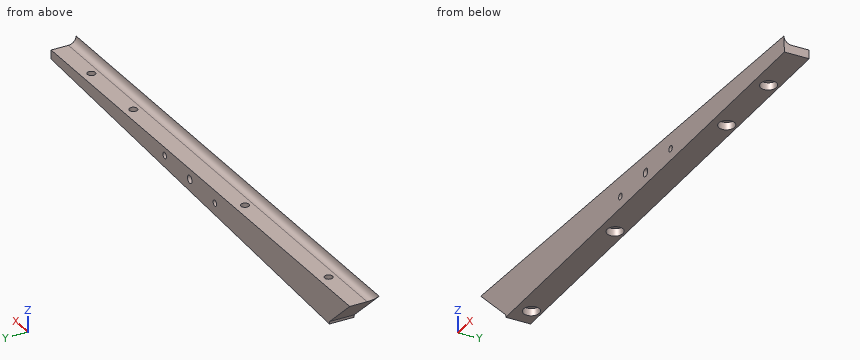
from build123d import *

# Parameters (mm, degrees)
CYLINDER033_R             = 1.6
CYLINDER033_DEPTH         = 100
CYLINDER034_R             = 1.25
CYLINDER034_DEPTH         = 100
CYLINDER035_R             = 1.25
CYLINDER035_DEPTH         = 100
FUSION027_PLACEMENT_ANGLE = 3.00002
CYLINDER012_R             = 3.2
CYLINDER012_DEPTH         = 3
CYLINDER013_R             = 1.6
CYLINDER013_DEPTH         = 30
CYLINDER014_R             = 3.2
CYLINDER014_DEPTH         = 3
CYLINDER015_R             = 1.6
CYLINDER015_DEPTH         = 30
CYLINDER016_R             = 3.2
CYLINDER016_DEPTH         = 3
CYLINDER017_R             = 1.6
CYLINDER017_DEPTH         = 30
CYLINDER011_R             = 3.2
CYLINDER011_DEPTH         = 3
CYLINDER010_R             = 1.6
CYLINDER010_DEPTH         = 30
BOX_W                     = 600
BOX_H                     = 10
BOX_DEPTH                 = 20
BOX_PLACEMENT_ANGLE       = 3
BOX001_W                  = 600
BOX001_H                  = 10
BOX001_DEPTH              = 20
BOX001_PLACEMENT_ANGLE    = 3
FILLET_R                  = 3
BOX003_W                  = 14
BOX003_H                  = 10
BOX003_DEPTH              = 27
BOX003_PLACEMENT_ANGLE    = 45
BOX002_W                  = 200
BOX002_H                  = 10
BOX002_DEPTH              = 17
CUT_PLACEMENT_ANGLE       = 2.999995


with BuildPart() as cylinder033:
    # Cylinder033 → Cylinder033 (new body)
    with BuildSketch(Plane(origin=(418, 0, 0), x_dir=(1, 0, 0), z_dir=(0, -1, 0))):
        Circle(CYLINDER033_R)
    extrude(amount=CYLINDER033_DEPTH)


with BuildPart() as cylinder034:
    # Cylinder034 → Cylinder034 (new body)
    with BuildSketch(Plane(origin=(436, 0, 0), x_dir=(1, 0, 0), z_dir=(0, -1, 0))):
        Circle(CYLINDER034_R)
    extrude(amount=CYLINDER034_DEPTH)


with BuildPart() as fusion027:
    # Cylinder035 → Cylinder035 (new body)
    with BuildSketch(Plane(origin=(400, 0, 0), x_dir=(1, 0, 0), z_dir=(0, -1, 0))):
        Circle(CYLINDER035_R)
    extrude(amount=CYLINDER035_DEPTH)

    # Fusion027: union Cylinder033, Cylinder034
    add(cylinder033.part)
    add(cylinder034.part)


with BuildPart() as fusion027_1:
    # Fusion027 placement: moved
    add(fusion027.part.moved(Location((83, 77, -26))).rotate(Axis((83, 77, -26), (0, -1, 0)), FUSION027_PLACEMENT_ANGLE))


with BuildPart() as cylinder012:
    # Cylinder012 → Cylinder012 (new body)
    with BuildSketch(Plane(origin=(578, 6, -35), x_dir=(1, 0, 0), z_dir=(0, 0, 1))):
        Circle(CYLINDER012_R)
    extrude(amount=CYLINDER012_DEPTH)


with BuildPart() as fusion013:
    # Cylinder013 → Cylinder013 (new body)
    with BuildSketch(Plane(origin=(578, 6, -35), x_dir=(1, 0, 0), z_dir=(0, 0, 1))):
        Circle(CYLINDER013_R)
    extrude(amount=CYLINDER013_DEPTH)

    # Fusion013: union Cylinder012
    add(cylinder012.part)


with BuildPart() as fusion013_1:
    # Fusion013 placement: moved
    add(fusion013.part.moved(Location((-170, 0, 21.1))))


with BuildPart() as cylinder014:
    # Cylinder014 → Cylinder014 (new body)
    with BuildSketch(Plane(origin=(578, 6, -35), x_dir=(1, 0, 0), z_dir=(0, 0, 1))):
        Circle(CYLINDER014_R)
    extrude(amount=CYLINDER014_DEPTH)


with BuildPart() as fusion014:
    # Cylinder015 → Cylinder015 (new body)
    with BuildSketch(Plane(origin=(578, 6, -35), x_dir=(1, 0, 0), z_dir=(0, 0, 1))):
        Circle(CYLINDER015_R)
    extrude(amount=CYLINDER015_DEPTH)

    # Fusion014: union Cylinder014
    add(cylinder014.part)


with BuildPart() as fusion014_1:
    # Fusion014 placement: moved
    add(fusion014.part.moved(Location((-110, 0, 24.3))))


with BuildPart() as cylinder016:
    # Cylinder016 → Cylinder016 (new body)
    with BuildSketch(Plane(origin=(578, 6, -35), x_dir=(1, 0, 0), z_dir=(0, 0, 1))):
        Circle(CYLINDER016_R)
    extrude(amount=CYLINDER016_DEPTH)


with BuildPart() as fusion015:
    # Cylinder017 → Cylinder017 (new body)
    with BuildSketch(Plane(origin=(578, 6, -35), x_dir=(1, 0, 0), z_dir=(0, 0, 1))):
        Circle(CYLINDER017_R)
    extrude(amount=CYLINDER017_DEPTH)

    # Fusion015: union Cylinder016
    add(cylinder016.part)


with BuildPart() as fusion015_1:
    # Fusion015 placement: moved
    add(fusion015.part.moved(Location((-30, 0, 28.5))))


with BuildPart() as cylinder011:
    # Cylinder011 → Cylinder011 (new body)
    with BuildSketch(Plane(origin=(578, 6, -35), x_dir=(1, 0, 0), z_dir=(0, 0, 1))):
        Circle(CYLINDER011_R)
    extrude(amount=CYLINDER011_DEPTH)


with BuildPart() as fusion035:
    # Cylinder010 → Cylinder010 (new body)
    with BuildSketch(Plane(origin=(578, 6, -35), x_dir=(1, 0, 0), z_dir=(0, 0, 1))):
        Circle(CYLINDER010_R)
    extrude(amount=CYLINDER010_DEPTH)

    # Fusion012: union Cylinder011
    add(cylinder011.part)


with BuildPart() as fusion035_1:
    # Fusion012 placement: moved
    add(fusion035.part.moved(Location((0, 0, 30))))

    # Fusion035: union Fusion013, Fusion014, Fusion015
    add(fusion013_1.part)
    add(fusion014_1.part)
    add(fusion015_1.part)


with BuildPart() as box:
    # Box → Box (new body)
    with BuildSketch(Plane.XY):
        with Locations((300, 5)):
            Rectangle(BOX_W, BOX_H)
    extrude(amount=BOX_DEPTH)


with BuildPart() as box_1:
    # Box placement: moved
    add(box.part.rotate(Axis((0, 0, 0), (0, 1, 0)), BOX_PLACEMENT_ANGLE))


with BuildPart() as fillet_body:
    # Box001 → Box001 (new body)
    with BuildSketch(Plane.XY):
        with Locations((300, 5)):
            Rectangle(BOX001_W, BOX001_H)
    extrude(amount=BOX001_DEPTH)


with BuildPart() as fillet_body_1:
    # Box001 placement: moved
    add(fillet_body.part.moved(Location((0, 52, 0))).rotate(Axis((0, 52, 0), (0, 1, 0)), BOX001_PLACEMENT_ANGLE))

    # Fusion: union Box
    add(box_1.part)

    # Fillet
    fillet_edges = [fillet_body_1.edges().sort_by_distance(p)[0] for p in [
        (300.63558, 62, 4.271804),
        (299.58886, 62, -15.700787),
        (299.58886, 0, -15.700787),
        (300.63558, 0, 4.271804),
    ]]
    fillet(fillet_edges, radius=FILLET_R)


with BuildPart() as box003:
    # Box003 → Box003 (new body)
    with BuildSketch(Plane.XY):
        with Locations((7, 5)):
            Rectangle(BOX003_W, BOX003_H)
    extrude(amount=BOX003_DEPTH)


with BuildPart() as box003_1:
    # Box003 placement: moved
    add(box003.part.moved(Location((400, 0, -35))).rotate(Axis((400, 0, -35), (0, -1, 0)), BOX003_PLACEMENT_ANGLE))


with BuildPart() as left_wheels_frame:
    # Box002 → Box002 (new body)
    with BuildSketch(Plane(origin=(399, 0, -35), x_dir=(1, 0, 0), z_dir=(0, 0, 1))):
        with Locations((100, 5)):
            Rectangle(BOX002_W, BOX002_H)
    extrude(amount=BOX002_DEPTH)

    # Fusion001: union Box003
    add(box003_1.part)

    # Cut: cut Fillet body
    add(fillet_body_1.part, mode=Mode.SUBTRACT)


with BuildPart() as left_wheels_frame_1:
    # Cut placement: moved
    add(left_wheels_frame.part.rotate(Axis((0, 0, 0), (0, -1, 0)), CUT_PLACEMENT_ANGLE))

    # Cut021: cut Fusion035
    add(fusion035_1.part, mode=Mode.SUBTRACT)

    # Cut022: cut Fusion027
    add(fusion027_1.part, mode=Mode.SUBTRACT)


with BuildPart() as left_wheels_frame_2:
    # Cut022 placement: moved
    add(left_wheels_frame_1.part.moved(Location((0, -10, 0))))


solid = left_wheels_frame_2.part
Verification items for the finished model (mm, model axes). Give positions to 0.01 mm unless a question says otherwise; leave off trailing zeros. Write each loop counter-clockwise with the first axis right and the second up, starting at its lowest first coordinate (ties: lowest second). Pieces come first, ordered by that corner, then holes.
(1) Cross-section at C-C (x = 477). Enter the section's corners in (y, z).
(2) Gauge pin test, flat ends, axial feed: pin 1 (4 mm diameter, centred on x = 468, y = -4, fed in from -Z); pin 2 (2 mm diameter, centred on x = 518.4, z = -3.18, fed in from -Y); pin 3 (5 mm diameter, centred on y = -8.5, z = -6.5, fed in from -X); pin 4 (3.5 mm diameter, centred on x = 548, y = -4, fed in from -Z). Record the tip position at first contact, or that the pin passes through.
(3) Cross-section at B-B (x = 567). Enter the section's corners in (y, z), plus the area to 3 significant figures.
(4) Cross-section at A-A (y = -4). State how many separate pieces and enclosed holes the cut face has, plus the area to 3 significant figures.
(5) Material ranges on line 1 (Y direction, x = 548, z = -2.15); line 2 (Y direction, x = 408, z = -13.1); line 3 (Z direction, x = 584, y = -1.75), recorded low to high.
Worked out:
1. outline: (-10, -10.05) - (0, -10.05) - (0, 0) - (-7, 0) arc R3 cw to (-10, 3) - close
2. pin 1: stops at z = -7.7
2. pin 2: passes through
2. pin 3: stops at x = 390.16
2. pin 4: stops at z = -3.5
3. outline: (-10, -5.33) - (0, -5.33) - (0, 0) - (-7, 0) arc R3 cw to (-10, 3) - close
3. area: 55.3 mm2
4. separate pieces: 5
4. enclosed holes: 3
4. area: 1,690 mm2
5. line 1: y = -10 to -5.6, -2.4 to 0
5. line 2: y = -10 to -7.2, -0.8 to 0
5. line 3: z = -4.44 to 0
